from build123d import *

# Parameters (mm, degrees)
F1_DEPTH = 7
F0_W     = 6
F0_H     = 5
F2_DEPTH = 25
F3_R     = 1.3748922144
F4_DEPTH = 25
F5_R     = 2.99999
F7_DEPTH = 25


# Not quite as in the source:
# - a fillet or chamfer is up to 0.001 mm smaller than in the source, because OpenCascade refuses the exact size


with BuildPart() as f1:
    # F0 (on Top) → F1 (new body)
    with BuildSketch(Plane.XY):
        with BuildLine():
            ThreePointArc((-1.690473047, 3.6252311481), (2.1491984334, 3.3735657833), (4, 0))
            ThreePointArc((4, 0), (2.1491984334, -3.3735657833), (-1.690473047, -3.6252311481))
            Line((-1.690473047, -3.6252311481), (-2.3244004396, -4.9846928287))
            ThreePointArc((-2.3244004396, -4.9846928287), (1.789005011, -5.2009096388), (4.8989794856, -2.5))
            ThreePointArc((4.8989794856, -2.5), (5.3476343915, -1.2856151892), (5.5, 0))
            ThreePointArc((5.5, 0), (5.3476343915, 1.2856151892), (4.8989794856, 2.5))
            ThreePointArc((4.8989794856, 2.5), (1.789005011, 5.2009096388), (-2.3244004396, 4.9846928287))
            Line((-2.3244004396, 4.9846928287), (-1.690473047, 3.6252311481))
        make_face()
        with BuildLine():
            Line((6.8989794856, 2.5), (4.8989794856, 2.5))
            ThreePointArc((4.8989794856, 2.5), (5.3476343915, 1.2856151892), (5.5, 0))
            ThreePointArc((5.5, 0), (5.3476343915, -1.2856151892), (4.8989794856, -2.5))
            Line((4.8989794856, -2.5), (6.8989794856, -2.5))
            Line((6.8989794856, -2.5), (6.8989794856, 2.5))
        make_face()
    extrude(amount=F1_DEPTH)

    # F0 (on Top) → F2 (join)
    with BuildSketch(Plane.XY):
        with Locations((9.8989794856, 0)):
            Rectangle(F0_W, F0_H)
    extrude(amount=F2_DEPTH)

    # F3 (on face) → F4 (cut)
    with BuildSketch(Plane.XZ.offset(2.5)):
        with Locations((9.8989794856, 21.5)):
            Circle(F3_R)
    extrude(amount=-F4_DEPTH, mode=Mode.SUBTRACT)

    # F5 (radius 3 in the source; OpenCascade refuses exactly that, so slightly less here)
    f5_edges = [f1.edges().sort_by_distance(p)[0] for p in [
        (12.898979, 0, 25),
        (6.898979, 0, 25),
    ]]
    fillet(f5_edges, radius=F5_R)

    # F6 (on face) → F7 (cut)
    with BuildSketch(Plane.XY.offset(7)):
        with BuildLine():
            Line((3.8729833462, -1), (6.8989794856, -1))
            Line((6.8989794856, -1), (6.8989794856, 1))
            Line((6.8989794856, 1), (3.8729833462, 1))
            ThreePointArc((3.8729833462, 1), (4, 0), (3.8729833462, -1))
        make_face()
    extrude(amount=-F7_DEPTH, mode=Mode.SUBTRACT)


solid = f1.part
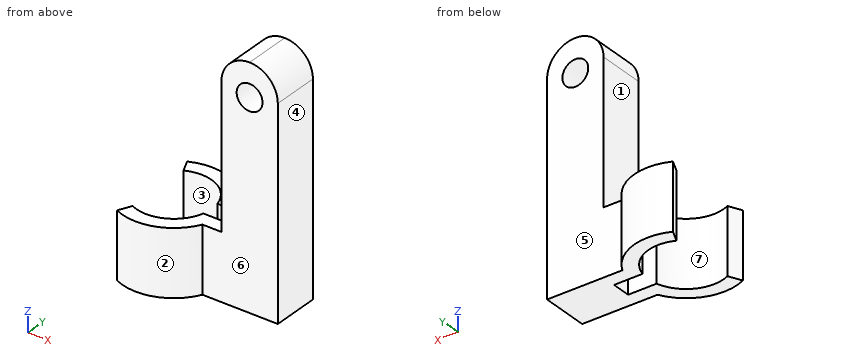
Build history of the part. All positions in model axes, mm. Face numbers are marked on the shaded views. A direction names the side the tool comes from. Give positions to 0.01 mm unless a question says otherwise; leave off trailing zeros. Order: outer loops, then holes, each group sorted by start corner. A loop starts at its lowest first (then second) coordinate and runs counter-clockwise, first axis right, second up. Notation, with made-up numbers: M -12,1 L 19,1 A26 ccw 19,18 Z; hole C -38,5 d9. An arc over 180 degrees is marked long. Put each result on its own line as item: value.
Item 1: Cut at C-C on z = 1.5. Write the cut outline in (x, y), then the cut area to 3 significant figures.
Results are:
outline: M -2.32,-4.98 A5.5 ccw 4.9,-2.5 L 12.9,-2.5 L 12.9,2.5 L 4.9,2.5 A5.5 ccw -2.32,4.98 L -1.69,3.63 A4 cw 3.87,1 L 6.9,1 L 6.9,-1 L 3.87,-1 A4 cw -1.69,-3.63 Z
area: 60.7 mm2
Item 2: Which spindle directions (+Z, -Z, +X, -X, +Y, -Y) get a long thin tool onto all of the face, cutting with end or side? Do the marked faces 5, 6 and 7. Say none if no direction does.
Results are:
face 5: +Z, -Z, +X, +Y
face 6: +Z, -Z, +X, -Y
face 7: +Z, -Z
Item 3: Wall check: probe 1 along Y at (x, z) = (8.75, 1.5); probe 2 along Z at (x, y) = (10, -0.25); probe 3 along X at (y, z) = (-0.25, 16.75). Give the ranges that are in metal, low to high.
Results are:
probe 1: -2.5 to 2.5
probe 2: 0 to 20.13, 22.87 to 25
probe 3: 6.9 to 12.9
Item 4: Cut at A-A on x = 6.25. Write the cut outline in (y, z), then the cut area to 3 significant figures.
Results are:
outline: M -2.5,0 L -1,0 L -1,7 L -2.5,7 Z; M 1,0 L 2.5,0 L 2.5,7 L 1,7 Z
area: 21.0 mm2
Item 5: Cut at D-D on y = 3. Write the cut outline in (x, z).
Results are:
outline: M 2.65,0 L 4.61,0 L 4.61,7 L 2.65,7 Z
Item 6: Cut at B-B on z = 21.5. Write the cut outline in (x, y), then the cut area to 3 significant figures.
Results are:
outline: M 6.9,-2.5 L 8.52,-2.5 L 8.52,2.5 L 6.9,2.5 Z; M 11.27,-2.5 L 12.9,-2.5 L 12.9,2.5 L 11.27,2.5 Z
area: 16.3 mm2
Item 7: Drop flat-ended pins along their axis: pin 1 Ø1.5 at (y, z) = (-2, 18) entering from -X; pin 2 Ø1 at (x, z) = (6.5, 20) entering from +Y; pin 3 Ø2.5 at (x, y) = (3, 3.5) entering from +Z; pin 4 Ø2 at (y, z) = (-4, 10) entering from +X. Give the stop position or say it passes through.
Results are:
pin 1: x = 6.9
pin 2: y = 2.5
pin 3: z = 7
pin 4: through
Item 8: Pull direction Y, two halves, no side cores. Call the marked faces 1, 2, 3 and 4: +Y half, -Y half, draft (parallel to the pull), parting line (faces both ways), or undercut.
Results are:
face 1: undercut
face 2: -Y half
face 3: undercut
face 4: draft
